The listing builds one solid part. Answer for the finished solid, in the listing's coordinates (mm). A direction names the side the tool comes from. Coordinates: 2 decimals unless noted, no trailing zeros. Write each loop counter-clockwise with the first axis right and the second up, starting at its lowest first coordinate (ties: lowest second). Pieces come first, ordered by that corner, then holes. Notation, with made-up numbers: M -2,12.25 L 32,12.25 A27 cw 32,33.25 Z; hole C 33,89.5 d7. An arc over 180 degrees is marked long. Put each result on its own line as item: value. Start each with the question number.
Autodesk Inventor part; units mm, degrees
ref_plane "for_body1_a_XY" through (9.525, 0, 0) normal (0, 1, 0) x (1, 0, 0)
ref_plane "for_body1_a_YZ" through (9.525, 0, 0) normal (1, 0, 0) x (0, 0, -1)
ref_plane "for_body1_a_ZX" through (9.525, 0, 0) normal (0, 0, -1) x (0, 1, 0)
sketch "Sketch_2" plane through (0, 0, 0) normal (0, 0, 1) x (1, 0, 0)
  line L0 (0, -2.86) -> (0, 2.86)
  line L1 (1.64, 2.86) -> (1.64, -2.86)
  line L2 (1.64, -2.86) -> (2.8575, -2.86)
  arc A0 (2.8575, -2.86) -> (3.175, -2.5425) centre (2.8575, -2.5425) ccw
  line L3 (3.175, -2.5425) -> (3.175, 2.5425)
  arc A1 (3.175, 2.5425) -> (2.8575, 2.86) centre (2.8575, 2.5425) ccw
  line L4 (2.8575, 2.86) -> (1.64, 2.86)
revolve "Revolution1" add sketch "Sketch_2" angle 360 about axis through (0, -2.86, 0) along (0, -1, 0)
sketch "Sketch_5" plane through (0, 2.86, 0) normal (0, 1, 0) x (1, 0, 0)
  arc A0 (0, 4.05) -> (0, -4.05) centre (0, 0) ccw
  line L0 (0, -4.05) -> (9.525, -4.05)
  arc A1 (9.525, -4.05) -> (9.525, 4.05) centre (9.525, 0) ccw
  line L1 (9.525, 4.05) -> (0, 4.05)
  circle A2 centre (9.525, 0) radius 1.64
  circle A3 centre (0, 0) radius 1.64
extrude "Extrusion1" add sketch "Sketch_5" along normal blind 1.3
sketch "Sketch_6" plane through (0, -2.86, 0) normal (0, 1, 0) x (1, 0, 0)
  arc A0 (0, 4.05) -> (0, -4.05) centre (0, 0) ccw
  line L0 (0, -4.05) -> (9.525, -4.05)
  arc A1 (9.525, -4.05) -> (9.525, 4.05) centre (9.525, 0) ccw
  line L1 (9.525, 4.05) -> (0, 4.05)
  circle A2 centre (9.525, 0) radius 1.64
  circle A3 centre (0, 0) radius 1.64
extrude "Extrusion2" add sketch "Sketch_6" against normal blind 1.3
sketch "Sketch_8" plane through (0, 0, 0) normal (0, 0, 1) x (1, 0, 0)
  line L0 (9.525, -2.86) -> (9.525, 2.86)
  line L1 (11.165, 2.86) -> (11.165, -2.86)
  line L2 (11.165, -2.86) -> (12.3825, -2.86)
  arc A0 (12.3825, -2.86) -> (12.7, -2.5425) centre (12.3825, -2.5425) ccw
  line L3 (12.7, -2.5425) -> (12.7, 2.5425)
  arc A1 (12.7, 2.5425) -> (12.3825, 2.86) centre (12.3825, 2.5425) ccw
  line L4 (12.3825, 2.86) -> (11.165, 2.86)
revolve "Revolution2" add sketch "Sketch_8" angle 360 about axis through (9.525, -2.86, 0) along (0, -1, 0)
ref_plane "for_body1_a_XY" through (9.525, 0, 0) normal (0, 1, 0) x (1, 0, 0)
ref_plane "for_body1_a_YZ" through (9.525, 0, 0) normal (1, 0, 0) x (0, 0, -1)
ref_plane "for_body1_a_ZX" through (9.525, 0, 0) normal (0, 0, -1) x (0, 1, 0)
ref_plane "to_dummy_XY" through (0, 0, 0) normal (0, 1, 0) x (1, 0, 0)
ref_plane "to_dummy_YZ" through (0, 0, 0) normal (1, 0, 0) x (0, 0, -1)
ref_plane "to_dummy_ZX" through (0, 0, 0) normal (0, 0, -1) x (0, 1, 0)
properties part number "06B - 1 RP - Body"
1) A cutting plane is placed at A-A on z = 0. State how many separate pieces and enclosed holes the cut face has, then the cut area to 3 significant figures.
2) Determine the mould class of faces 3 (the face through (7.887, 0.058, -0.072)), 4 (the face through (5, 4, -4.05)), 5 (the face through (12.458, 0.036, 1.216)) for opening direction Z: +Z half, -Z half, draft (parallel to the pull), parting line (faces both ways), or undercut.
3) For faces 1 (the face through (-0.69, 0.04, 3.1)), 2 (the face through (5, -4.16, 0)), determine the directions among +Z, -Z, +X, -X, +Y, -Y from which every point of the face is accessible in a straight line to the end or side of a thin tool.
4) Given pin 1 Ø1 at (y, z) = (2.5, 3) entering from +X; pin 2 Ø1 at (x, y) = (2, 1.5) entering from -Z; pin 3 Ø3 at (y, z) = (0, 2.5) entering from -X, each flat-ended and moving along its own axis, determine where each tip first touches the part or whether it passes through.
5) Straight lines are drawn through the part: probe 1 along Y at (x, z) = (7.25, 2.75); probe 2 along Z at (x, y) = (0, -2) (3 decimals); probe 3 along X at (y, z) = (-0.75, 0.5). For each, find the intervals that lie inside material, in ascending order.
6) A cutting plane is placed at B-B on y = -1. Write down the section's boundary in (x, z) (3 decimals).
Answers follow:
1. separate pieces: 3
1. enclosed holes: 1
1. area: 63.7 mm²
2. face 3: undercut
2. face 4: -Z half
2. face 5: parting line
3. face 1: none
3. face 2: +Z, -Z, +X, -X, -Y
4. pin 1: stops at x = 12.59
4. pin 2: stops at z = -2.8
4. pin 3: stops at x = -3.01
5. probe 1: y = -4.16 to -2.86, 2.86 to 4.16
5. probe 2: z = -3.175 to -1.64, 1.64 to 3.175
5. probe 3: x = -3.14 to -1.56, 1.56 to 3.14, 6.39 to 7.96, 11.09 to 12.66
6. outline: C 0,0 d6.35; C 9.525,0 d6.35; hole C 0,0 d3.28; hole C 9.525,0 d3.28
